Geometry check sheet. Reference: drawing and pictorial views, mm from the part's lowest x, y, z. A direction names the side the tool comes from. Round coordinates to 2 decimals unless told otherwise and drop trailing zeros. Order: outer loops, then holes, each group sorted by start corner. A loop starts at its lowest first (then second) coordinate and runs counter-clockwise, first axis right, second up.
(1) Thickness scan on probe 1 along Z at (x, y) = (23.5, 6); probe 2 along Y at (x, z) = (20.75, 5); probe 3 along Y at (x, z) = (19, 11.25). Record the ranges inside material, lowest first.
(2) Sectioned sample at D-D, the plane x = 27. Enter the section's corners in (y, z).
(3) Mould release check, pull along X, two halves, no side actions. Record for the marked faces 3, 4, 5 and 6: released by +X, released by -X, zero draft, split by the parting line, or undercut.
(4) Sectioned sample at B-B, the plane x = 15.75. Enter the section's corners in (y, z), and give its area (3 significant figures).
(5) Depth check by flat-ended pin: pin 1 (2 mm diameter, centred on x = 11, z = 3, fed in from +Y); pin 2 (3 mm diameter, centred on y = 25.5, z = 6, fed in from -X); pin 3 (1.5 mm diameter, centred on x = 26.5, z = 6, fed in from +Y); pin 4 (11.5 mm diameter, centred on x = 14.94, y = 17.25, fed in from +Z). Enter the tip coordinate at first touch or a pass-through.
(6) Tool access check on the marked faces 1 and 2. Record the directions out of +Z, -Z, +X, -X, +Y, -Y that give a thin tool (end or side, any length) a straight path to the whole face; none if there is none.
(7) Sectioned sample at C-C, the plane z = 18.75. Enter the section's corners in (x, y) (3 decimals).
(8) Sectioned sample at A-A, the plane y = 17.25. Enter the section's corners in (x, z).
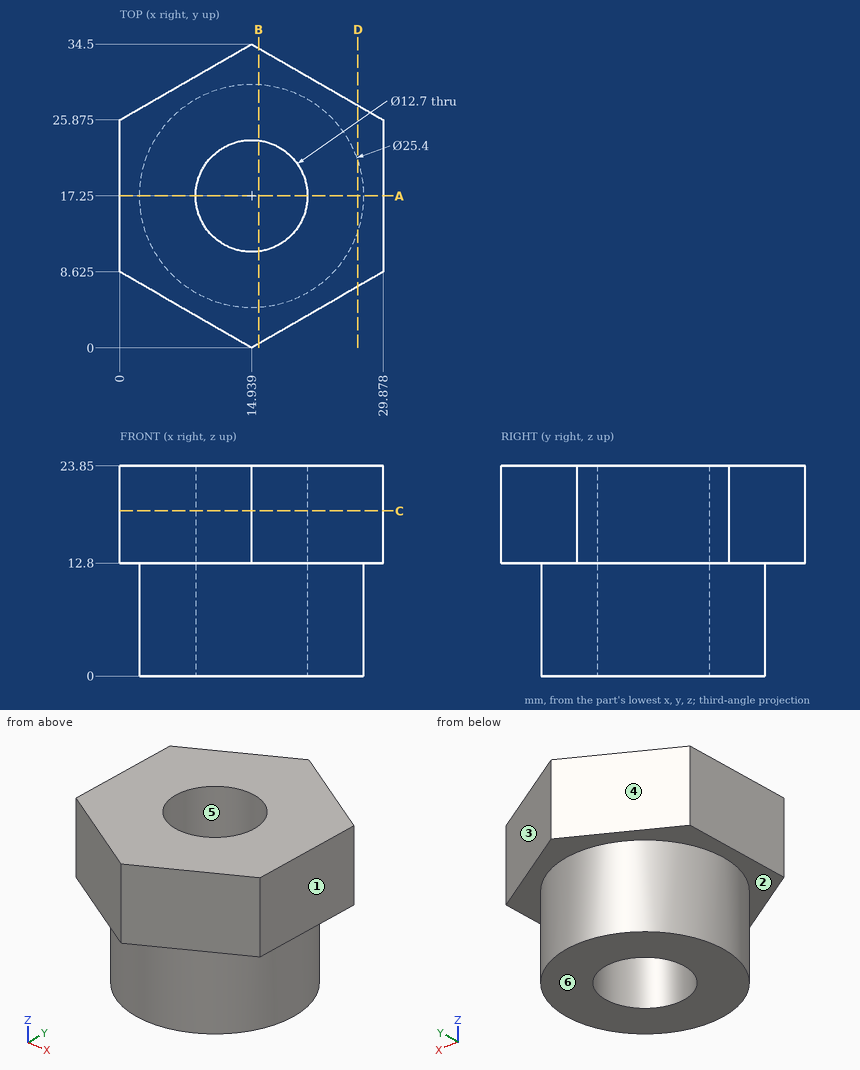
Derived:
1. probe 1: z = 12.8 to 23.85
1. probe 2: y = 5.96 to 14.69, 19.81 to 28.54
1. probe 3: y = 5.22 to 12.37, 22.13 to 29.28
2. outline: (6.96, 12.8) - (13.27, 12.8) - (13.27, 0) - (21.23, 0) - (21.23, 12.8) - (27.54, 12.8) - (27.54, 23.85) - (6.96, 23.85) - close
3. face 3: released by +X
3. face 4: released by -X
3. face 5: undercut
3. face 6: zero draft
4. outline: (0.47, 12.8) - (4.58, 12.8) - (4.58, 0) - (10.95, 0) - (10.95, 23.85) - (0.47, 23.85) - close; (23.55, 0) - (29.92, 0) - (29.92, 12.8) - (34.03, 12.8) - (34.03, 23.85) - (23.55, 23.85) - close
4. area: 395 mm2
5. pin 1: stops at y = 29.61
5. pin 2: stops at x = 4.18
5. pin 3: stops at y = 23.91
5. pin 4: passes through
6. face 1: +Z, -Z, +X, +Y, -Y
6. face 2: -Z
7. outline: (0, 8.625) - (14.939, 0) - (29.878, 8.625) - (29.878, 25.875) - (14.939, 34.5) - (0, 25.875) - close; hole circle Ø12.7 at (14.939, 17.25)
8. outline: (0, 12.8) - (2.24, 12.8) - (2.24, 0) - (8.59, 0) - (8.59, 23.85) - (0, 23.85) - close; (21.29, 0) - (27.64, 0) - (27.64, 12.8) - (29.88, 12.8) - (29.88, 23.85) - (21.29, 23.85) - close
